Can you work these out from the model? Positions are in its coordinate system, mm. A direction names the side the tool comes from. Coordinates: 2 decimals unless noted, no trailing zeros. Loops run counter-clockwise (first coordinate to the right, second up) from the corner with the lowest first, then second, coordinate; pieces in that order, holes last. Notation, with made-up numbers: M 74.25,-24 L 120.25,-24 A21 cw 120.25,-19 Z; hole C 64.25,10 d6. An arc over 180 degrees is marked long. Answer as a JSON object with one key per item and string values. Group by question number.
Item 1: We'd pull the mould along Z, two halves only. Please class faces 1 (the flat face through (-1, 0, 9)), 2 (the cylindrical face through (1.281, 0.065, 22.994)), 3 (the flat face through (76, -2.625, 15)): +Z half, -Z half, draft (parallel to the pull), parting line (faces both ways), or undercut.
Item 2: Suppose I cut it at B-B (z = 13.75). Write out the boundary of the cut face in (x, y) (3 decimals), then the cut area to 3 significant figures.
Item 3: I'm going to push a flat-ended pin straight in: pin 1 Ø3 at (x, z) = (77, 16) entering from -Y (3 decimals). Where does the tip first touch, or does it pass through?
Item 4: Suppose I cut it at C-C (z = 22.25). Write out the boundary of the cut face in (x, y) (3 decimals).
Item 5: If I drill on line 1 (X direction, y = -4, z = 16); line 2 (X direction, y = 1.5, z = 17.75); line 3 (X direction, y = -1.25, z = 19.75), over which ranges is the centre line in solid material (lowest first)?
Item 6: Which directions (+Z, -Z, +X, -X, +Y, -Y) give clear straight access to the entire face, cutting with the end or side of a thin tool? Please do faces 4 (the cylindrical face through (63.6, -3.89, 19.83)), 5 (the cylindrical face through (106.594, 0.065, 23.119)).
Item 7: Suppose I cut it at A-A (x = 71). Write out the boundary of the cut face in (y, z) (3 decimals), then the cut area to 3 significant figures.
```python
from build123d import *

# Parameters (mm, degrees)
F0_W     = 110
F0_H     = 25.4
F1_DEPTH = 4.625
F3_DEPTH = 2
F4_R     = 0.5
F5_R     = 8


with BuildPart() as f1:
    # F0 (on Front) → F1 (new body, symmetric)
    with BuildSketch(Plane.XZ):
        with Locations((54, 12.7)):
            Rectangle(F0_W, F0_H)
    extrude(amount=F1_DEPTH, both=True)

    # F2 (on face) → F3 (cut)
    with BuildSketch(Plane.XZ.offset(4.625)):
        with BuildLine():
            ThreePointArc((20, 11), (20.585786, 9.585786), (22, 9))
            Line((22, 9), (44, 9))
            ThreePointArc((44, 9), (45.414214, 9.585786), (46, 11))
            Line((46, 11), (46, 18.4))
            ThreePointArc((46, 18.4), (45.414214, 19.814214), (44, 20.4))
            Line((44, 20.4), (22, 20.4))
            ThreePointArc((22, 20.4), (20.585786, 19.814214), (20, 18.4))
            Line((20, 18.4), (20, 11))
        make_face()
        with BuildLine():
            Line((87, 20.4), (65, 20.4))
            ThreePointArc((65, 20.4), (63.585786, 19.814214), (63, 18.4))
            Line((63, 18.4), (63, 11))
            ThreePointArc((63, 11), (63.585786, 9.585786), (65, 9))
            Line((65, 9), (87, 9))
            ThreePointArc((87, 9), (88.414214, 9.585786), (89, 11))
            Line((89, 11), (89, 18.4))
            ThreePointArc((89, 18.4), (88.414214, 19.814214), (87, 20.4))
        make_face()
    extrude(amount=-F3_DEPTH, mode=Mode.SUBTRACT)

    # F4
    f4_edges = [f1.edges().sort_by_distance(p)[0] for p in [
        (89, -2.625, 14.7),
        (46, -2.625, 14.7),
    ]]
    fillet(f4_edges, radius=F4_R)

    # F5
    f5_edges = [f1.edges().sort_by_distance(p)[0] for p in [
        (109, 0, 25.4),
        (-1, 0, 25.4),
    ]]
    fillet(f5_edges, radius=F5_R)


solid = f1.part
```
From the geometry:
{
 "1": {"face 1": "draft", "face 2": "+Z half", "face 3": "undercut"},
 "2": {"outline": "M -1,-4.625 L 20,-4.625 L 20,-3.125 A0.5 cw 20.5,-2.625 L 45.5,-2.625 A0.5 cw 46,-3.125 L 46,-4.625 L 63,-4.625 L 63,-3.125 A0.5 cw 63.5,-2.625 L 88.5,-2.625 A0.5 cw 89,-3.125 L 89,-4.625 L 109,-4.625 L 109,4.625 L -1,4.625 Z", "area": "914 mm2"},
 "3": {"pin 1": "y = -2.625"},
 "4": {"outline": "M 0.638,-4.625 L 107.362,-4.625 L 107.362,4.625 L 0.638,4.625 Z"},
 "5": {"line 1": "-1 to 20, 46 to 63, 89 to 109", "line 2": "-0.99 to 108.99", "line 3": "-0.65 to 108.65"},
 "6": {"face 4": "-Y", "face 5": "+Z, +X, +Y, -Y"},
 "7": {"outline": "M -4.625,0 L 4.625,0 L 4.625,25.4 L -4.625,25.4 L -4.625,20.4 L -3.125,20.4 A0.5 cw -2.625,19.9 L -2.625,9.5 A0.5 cw -3.125,9 L -4.625,9 Z", "area": "212 mm2"}
}
